Geometry: see drawing. Coordinates: mm, zero at the bounding-box minimum. Round coordinates to 2 decimals unless told otherwise and drop trailing zeros. Write each loop counter-clockwise with the first axis right and the second up, starting at its lowest first coordinate (ties: lowest second). Pieces come first, ordered by that corner, then holes. Notation, with made-up numbers: (69.25, 73.25) - (82.25, 73.25) arc R14 ccw to (82.25, 92.25) - close; hole circle Ø11 at (40.5, 86). An arc over 180 degrees is marked (long way). One line per item, written item: value. Start each with the question number.
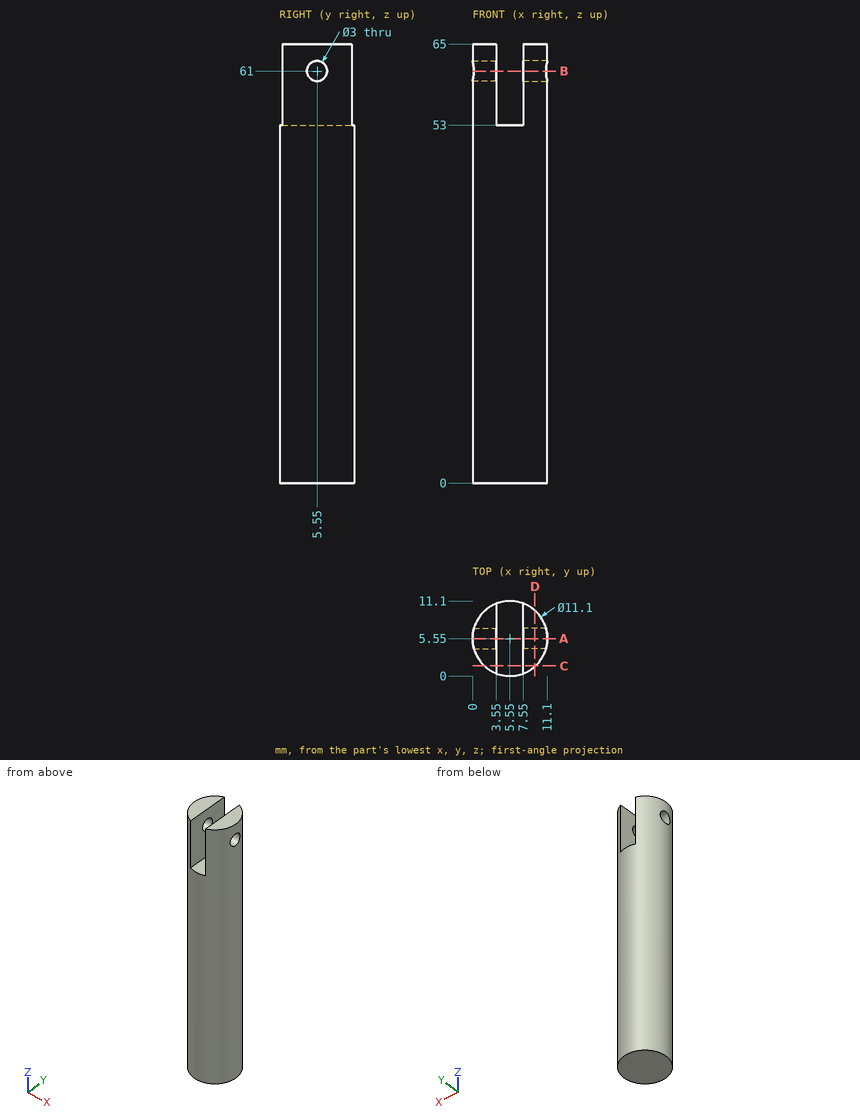
Q1. Cut plane A-A, the plane y = 5.55. Output: boundary loops of the cut face in (x, z).
Q2. Material intervals for probe 1 along Z at (x, y) = (5.25, 9.5); probe 2 along Y at (x, z) = (8.8, 61); probe 3 along Y at (x, z) = (9.5, 61), sorted ascending. Write a range as from..to.
Q3. Cut plane C-C, the plane y = 1.5. Output: boundary loops of the cut face in (x, z).
Q4. Cut plane D-D, the plane x = 9.25. Output: boundary loops of the cut face in (y, z), and give its area (3 significant figures).
Q5. Cut plane B-B, the plane z = 61. Output: boundary loops of the cut face in (x, y).
Q6. Contact query for flat-ended pins moving along their axis: pin 1 Ø1.5 at (x, z) = (2.5, 22) entering from -Y; pin 2 Ø1 at (y, z) = (9, 12.5) entering from +X; pin 3 Ø6 at (x, z) = (1, 35) entering from -Y. Output: stop coordinate, or through.
A:
1. outline: (0, 0) - (11.1, 0) - (11.1, 59.5) - (7.55, 59.5) - (7.55, 53) - (3.55, 53) - (3.55, 59.5) - (0, 59.5) - close; (0, 62.5) - (3.55, 62.5) - (3.55, 65) - (0, 65) - close; (7.55, 62.5) - (11.1, 62.5) - (11.1, 65) - (7.55, 65) - close
2. probe 1: z = 0..53
2. probe 2: y = 1.05..4.05, 7.05..10.05
2. probe 3: y = 1.65..4.05, 7.05..9.45
3. outline: (1.76, 0) - (9.34, 0) - (9.34, 65) - (7.55, 65) - (7.55, 53) - (3.55, 53) - (3.55, 65) - (1.76, 65) - close
4. outline: (1.41, 0) - (9.69, 0) - (9.69, 65) - (1.41, 65) - close; hole circle Ø3 at (5.55, 61)
4. area: 531 mm²
5. outline: (0.21, 4.05) arc R5.55 ccw to (3.55, 0.37) - (3.55, 4.05) - close; (0.21, 7.05) - (3.55, 7.05) - (3.55, 10.73) arc R5.55 ccw to start; (7.55, 0.37) arc R5.55 ccw to (10.89, 4.05) - (7.55, 4.05) - close; (7.55, 7.05) - (10.89, 7.05) arc R5.55 ccw to (7.55, 10.73) - close
6. pin 1: stops at y = 0.5
6. pin 2: stops at x = 10.25
6. pin 3: stops at y = 0.22
